Geometry: final body of the model. Coordinates: model frame, mm. Face numbers are marked on the shaded views. A direction names the side the tool comes from. Give positions to 0.01 mm unless a question says otherwise; leave off trailing zeros. Order: outer loops, then holes, each group sorted by start corner. A loop starts at its lowest first (then second) coordinate and runs counter-clockwise, first axis right, second up. Notation, with made-up numbers: M 69,6 L 79,6 A13 cw 79,12 Z; hole C 14,42 d1. An arc over 180 degrees is marked long. Use CSV: the item, a comma, the result in double quotes.
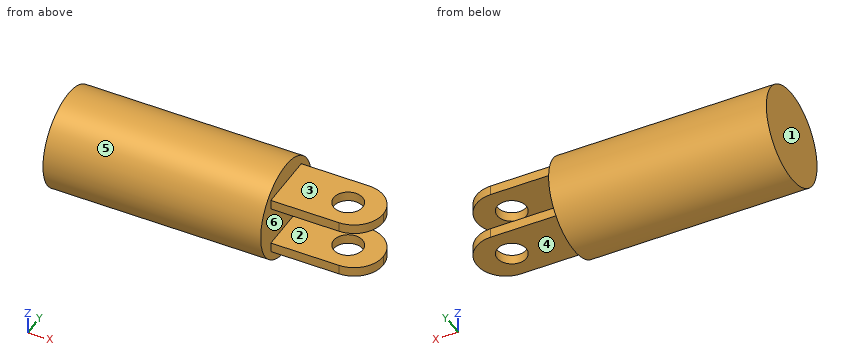
Autodesk Inventor part; units mm, degrees
ref_plane "YZ Plane" through (0, 0, 0) normal (1, 0, 0) x (0, 1, 0)
ref_plane "XZ Plane" through (0, 0, 0) normal (0, 1, 0) x (-1, 0, 0)
ref_plane "XY Plane" through (0, 0, 0) normal (0, 0, 1) x (1, 0, 0)
sketch "Schizzo1" plane through (0, 0, 0) normal (1, 0, 0) x (0, 1, 0)
  circle A0 centre (0, 0) radius 5
  dimension "d0" = 10
extrude "Estrusione1" add sketch "Schizzo1" along normal blind 22.39
sketch "Schizzo2" plane through (22.39, 0, 0) normal (1, 0, 0) x (0, 0, -1)
  line L0 (-3, 3) -> (3, 3)
  line L1 (3, 3) -> (3, -3)
  line L2 (3, -3) -> (-3, -3)
  line L3 (-3, -3) -> (-3, 3)
  line L4 (-3, 3) -> (3, -3) construction
  line L5 (3, 3) -> (-3, -3) construction
  point P0 (0, 0)
  point P1 (0, 0)
  point P2 (0, 0)
  dimension "d3" = 6
  dimension "d4" = 6
extrude "Estrusione2" add sketch "Schizzo2" along normal blind 10
sketch "Schizzo5" plane through (22.39, 3, 3) normal (0, 1, 0) x (1, 0, 0)
  line L0 (0, -2) -> (0, 8)
  line L1 (10, 5) -> (0, 5)
  line L2 (0, 5) -> (0, 1)
  line L3 (0, 1) -> (10, 1)
  line L4 (10, 1) -> (10, 5)
  line L5 (10, 6) -> (10, 0)
  point P0 (-22.39, 3)
  point P1 (10, 3)
  point P2 (0, 5)
  dimension "d19" = 4
extrude "Estrusione5" cut sketch "Schizzo5" against normal blind 15
sketch "Schizzo6" plane through (22.39, -3, 3) normal (0, 0, 1) x (1, 0, 0)
  circle A0 centre (6.39, 3) radius 1.5
  line L0 (0, 0) -> (10, 0)
  line L1 (10, 6) -> (10, 0)
  line L2 (0, -2) -> (0, 8)
  point P0 (-22.39, 3)
  dimension "d22" = 3
  dimension "d24" = 3
  dimension "d28" = 6.39
extrude "Estrusione6" cut sketch "Schizzo6" against normal blind 15
fillet "Raccordo2" radius 3 4 edges at (32.39, 3, 2.5) (32.39, 3, -2.5) (32.39, -3, -2.5) (32.39, -3, 2.5)
properties part number "pistone" material "Titanio"
1. Pin query (flat end, axial travel): pin 1 Ø0.8 at (x, z) = (24.5, 2.5) entering from +Y; pin 2 Ø0.8 at (x, z) = (26, 2.5) entering from -Y; pin 3 Ø4 at (y, z) = (3.5, 3) entering from +X; pin 4 Ø2.5 at (x, y) = (28.78, 0) entering from +Z. Return the tip coordinate at first contact, or that it passes through.
Answer:
pin 1,"y = 3"
pin 2,"y = -3"
pin 3,"x = 31.99"
pin 4,"through"
2. Section A-A, the plane x = 28.78. Return the cut outline in (y, z).
Answer:
outline,"M -3,-3 L -1.5,-3 L -1.5,-2 L -3,-2 Z; M -3,2 L -1.5,2 L -1.5,3 L -3,3 Z; M 1.5,-3 L 3,-3 L 3,-2 L 1.5,-2 Z; M 1.5,2 L 3,2 L 3,3 L 1.5,3 Z"
3. Section B-B, the plane y = 2. Return the cut outline in (x, z).
Answer:
outline,"M 0,-4.58 L 22.39,-4.58 L 22.39,-3 L 31.63,-3 L 31.63,-2 L 22.39,-2 L 22.39,2 L 31.63,2 L 31.63,3 L 22.39,3 L 22.39,4.58 L 0,4.58 Z"
4. Pull-direction query (Z, two-part tool) for the marked faces 4, 5 and 6; classes: +Z half, -Z half, draft (parallel to the pull), parting line (faces both ways), or undercut.
Answer:
face 4,"-Z half"
face 5,"parting line"
face 6,"undercut"
5. Line query: line 1 (Y direction, x = 28.78, z = 2.4); line 2 (Z direction, x = 24, y = -2.25); line 3 (X direction, y = 1.5, z = 1.25). Output: solid intervals per line, ascending.
Answer:
line 1,"-3 to -1.5, 1.5 to 3"
line 2,"-3 to -2, 2 to 3"
line 3,"0 to 22.39"
6. Section C-C, the plane z = 0. Return the cut outline in (x, y).
Answer:
outline,"M 0,-5 L 22.39,-5 L 22.39,5 L 0,5 Z"
7. Reachability of the marked faces 1, 2 and 3 from +Z, -Z, +X, -X, +Y, -Y: full face, straight path, thin tool, end or side. Return the list, or none.
Answer:
face 1,"+Z, -Z, -X, +Y, -Y"
face 2,"+X, +Y, -Y"
face 3,"+Z, +X, +Y, -Y"
8. Section D-D, the plane x = 17. Return the cut outline in (y, z), plus the area to 3 significant figures.
Answer:
outline,"C 0,0 d10"
area,"78.5 mm2"
